The drawing under review shows one solid part. Ordinate dimensions are in mm from its lowest x, y, z. A direction names the side the tool comes from. Give positions to 0.01 mm unless a question says otherwise; leave off trailing zeros. Write each loop counter-clockwise with the first axis right and the second up, starting at its lowest first coordinate (ties: lowest second). Pieces come first, ordered by that corner, then holes. Notation, with made-up numbers: (-40, 81) -> (-9, 81) arc R25 ccw to (-9, 119) -> close; hole circle Ø5 at (17, 27.5). An arc over 180 degrees is marked (long way). Answer as a JSON object with one key per item and string values.
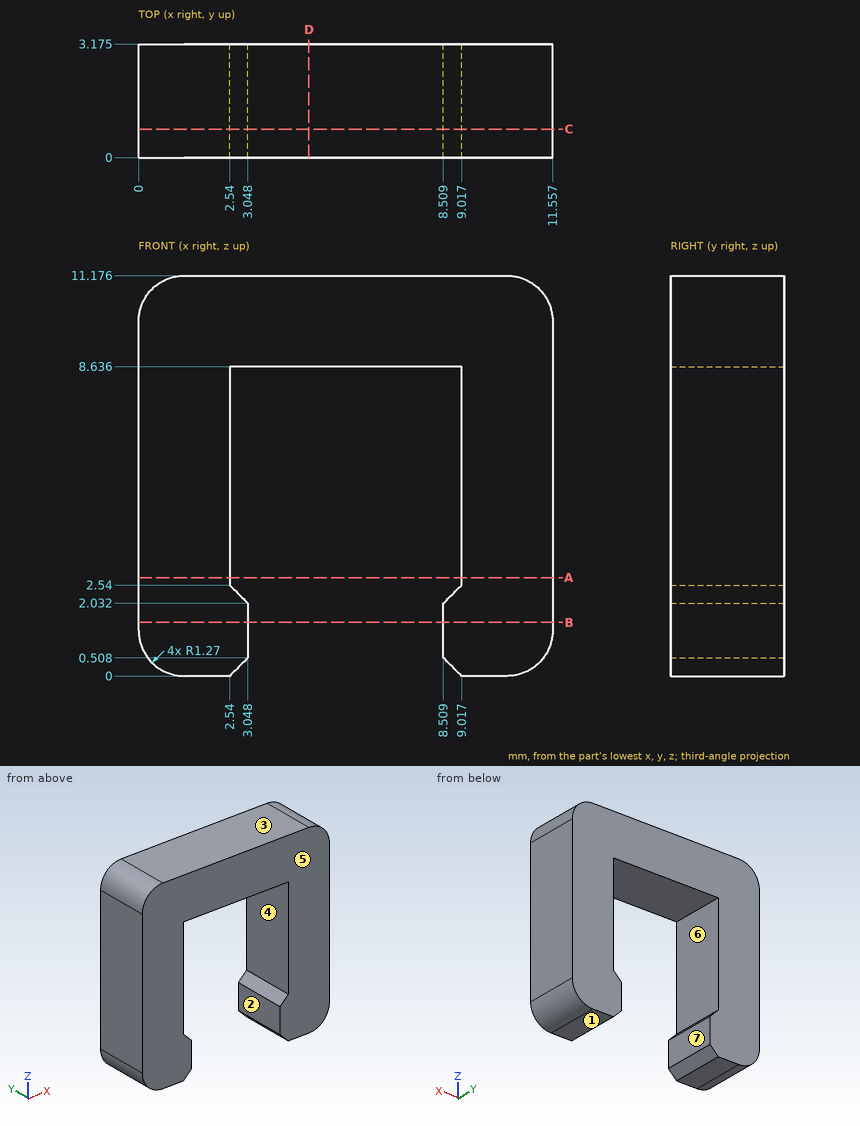
(1) For line 1 along X through (y, z) = (2.35, 8.5); line 2 along X through (y, z) = (2.05, 2); line 3 along Z through (x, y) = (7.25, 0.8), list the stretches that pass through material, from the lowest coordinate up.
Here are the results:
{"line 1": "x = 0 to 2.54, 9.02 to 11.56", "line 2": "x = 0 to 3.05, 8.51 to 11.56", "line 3": "z = 8.64 to 11.18"}
(2) We need section A-A, the plane z = 2.75. State the section outline as (x, y) points (3 decimals).
Here are the results:
{"outline": "(0, 0) -> (2.54, 0) -> (2.54, 3.175) -> (0, 3.175) -> close; (9.017, 0) -> (11.557, 0) -> (11.557, 3.175) -> (9.017, 3.175) -> close"}
(3) We need section D-D, the plane x = 4.75. State the section outline as (y, z) points (3 decimals), then the cut area to 3 significant figures.
Here are the results:
{"outline": "(0, 8.636) -> (3.175, 8.636) -> (3.175, 11.176) -> (0, 11.176) -> close", "area": "8.06 mm²"}
(4) The part is to be moulded in two halves that separate along Z. For the marked faces 1, 2, 3 and 4, say which applies: +Z half, -Z half, draft (parallel to the pull), parting line (faces both ways), or undercut.
Here are the results:
{"face 1": "-Z half", "face 2": "draft", "face 3": "+Z half", "face 4": "undercut"}
(5) We need section B-B, the plane z = 1.5. State the section outline as (x, y) points (3 decimals), then the cut area to 3 significant figures.
Here are the results:
{"outline": "(0, 0) -> (3.048, 0) -> (3.048, 3.175) -> (0, 3.175) -> close; (8.509, 0) -> (11.557, 0) -> (11.557, 3.175) -> (8.509, 3.175) -> close", "area": "19.4 mm²"}
(6) We need section C-C, the plane y = 0.8. State the section outline as (x, z) points.
Here are the results:
{"outline": "(0, 1.27) arc R1.27 ccw to (1.27, 0) -> (2.54, 0) -> (3.05, 0.51) -> (3.05, 2.03) -> (2.54, 2.54) -> (2.54, 8.64) -> (9.02, 8.64) -> (9.02, 2.54) -> (8.51, 2.03) -> (8.51, 0.51) -> (9.02, 0) -> (10.29, 0) arc R1.27 ccw to (11.56, 1.27) -> (11.56, 9.91) arc R1.27 ccw to (10.29, 11.18) -> (1.27, 11.18) arc R1.27 ccw to (0, 9.91) -> close"}
(7) Clearance check with a flat-ended pin moving along its axis: pin 1 (0.5 mm diameter, centred on y = 2, z = 1, fed in from -X). State where the tip first meets the part, or that it passes through.
Here are the results:
{"pin 1": "stops at x = 0"}
(8) For the marked faces 5, 6 and 7, list the 3-axis set-ups (+Z, -Z, +X, -X, +Y, -Y) from which the entire face can be reached by the end or side of a thin tool; tool diameter is ignored.
Here are the results:
{"face 5": "+Z, -Z, +X, -X, -Y", "face 6": "+Y, -Y", "face 7": "-Z, +Y, -Y"}
